Source: CAD feature listing. Evaluate the final solid. Frame: model axes, mm. Round coordinates to 2 decimals unless told otherwise and drop trailing zeros. Loops run counter-clockwise (first coordinate to the right, second up) from the corner with the lowest first, then second, coordinate; pieces in that order, holes last. Notation, with made-up numbers: (23.5, 19) - (56.5, 19) arc R13 ccw to (56.5, 27) - close; hole circle Ø9 at (-13.75, 86.5). An arc over 180 degrees is marked (long way). One line per question, with ' | ' between items. Start each with the question number.
1. Cut plane B-B (z = 12.75). Return loops of the section in (x, y), then the cut area to 3 significant figures.
2. Mould query, pull axis Z, two halves, no side actions, for faces 1 (the cylindrical face through (32, 1, 16)), 2 (the flat face through (0, 1, 13)), 3 (the flat face through (38, 1, 25.5)). Classes: pulls with the +Z half, pulls with the -Z half, needs draft (parallel to the pull), parting line crosses it, or undercut.
3. Ray query, line 1 (X direction, y = 1, z = 12.75); line 2 (Z direction, x = 30.7, y = 1); line 3 (X direction, y = 0.55, z = 11.25). Return the intervals inside material, ascending.
4. Cut plane A-A (x = 30.7). Return loops of the section in (y, z), then the cut area to 4 significant figures.
5. Cut plane C-C (y = 0.55). Return loops of the section in (x, z), then the cut area to 3 significant figures.
Autodesk Inventor part; units mm, degrees
ref_plane "YZ Plane" through (0, 0, 0) normal (1, 0, 0) x (0, 1, 0)
ref_plane "XZ Plane" through (0, 0, 0) normal (0, 1, 0) x (-1, 0, 0)
ref_plane "XY Plane" through (0, 0, 0) normal (0, 0, 1) x (1, 0, 0)
sketch "Sketch1" plane through (0, 0, 0) normal (0, 1, 0) x (-1, 0, 0)
  line L0 (0, 0) -> (-75.4, 0)
  line L1 (-75.4, 0) -> (-75.4, 25.5)
  line L2 (-75.4, 25.5) -> (0, 25.5)
  line L3 (0, 25.5) -> (0, 0)
  dimension "d0" = 75.4
  dimension "d1" = 25.5
extrude "Extrusion1" add sketch "Sketch1" along normal blind 1.3
sketch "Sketch6" plane through (0, 1.3, 0) normal (0, 1, 0) x (1, 0, 0)
  line L0 (75.4, 0) -> (0, 0)
  line L1 (0, 0) -> (0, -25.5)
  line L2 (0, -25.5) -> (75.4, -25.5)
  line L3 (75.4, -25.5) -> (75.4, 0)
  circle A0 centre (30.7, -12.75) radius 3.5
  dimension "d20" = 7
  dimension "d24" = 30.7
extrude "Extrusion6" cut sketch "Sketch6" against normal blind 10 contours A0
properties part number "00_Microscopeslide"
Answers follow:
1) outline: (0, 0) - (27.2, 0) - (27.2, 1.3) - (0, 1.3) - close; (34.2, 0) - (75.4, 0) - (75.4, 1.3) - (34.2, 1.3) - close | area: 88.9 mm2
2) face 1: undercut | face 2: needs draft | face 3: pulls with the +Z half
3) line 1: x = 0 to 27.2, 34.2 to 75.4 | line 2: z = 0 to 9.25, 16.25 to 25.5 | line 3: x = 0 to 27.54, 33.86 to 75.4
4) outline: (0, 0) - (1.3, 0) - (1.3, 9.25) - (0, 9.25) - close; (0, 16.25) - (1.3, 16.25) - (1.3, 25.5) - (0, 25.5) - close | area: 24.05 mm2
5) outline: (0, 0) - (75.4, 0) - (75.4, 25.5) - (0, 25.5) - close; hole circle Ø7 at (30.7, 12.75) | area: 1,880 mm2
